Geometry check sheet. Reference: the model listing, model coordinates, mm. Give positions to 0.01 mm unless a question says otherwise; leave off trailing zeros. Write each loop counter-clockwise with the first axis right and the second up, starting at its lowest first coordinate (ties: lowest second). Pieces come first, ordered by that corner, then holes. Notation, with made-up numbers: (66.5, -29) - (116.5, -29) arc R21 cw to (116.5, -25) - close; hole circle Ø11 at (2.5, -10). An arc over 180 degrees is marked (long way). Use a Markdown table: item, result.
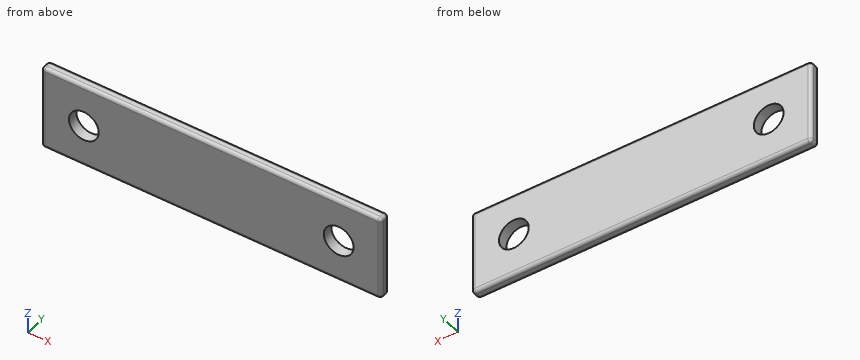
Autodesk Inventor part; units mm, degrees
ref_plane "YZ Plane" through (0, 0, 0) normal (1, 0, 0) x (0, 1, 0)
ref_plane "XZ Plane" through (0, 0, 0) normal (0, 1, 0) x (-1, 0, 0)
ref_plane "XY Plane" through (0, 0, 0) normal (0, 0, 1) x (1, 0, 0)
sketch "Sketch1" plane through (0, 0, 0) normal (0, 1, 0) x (-1, 0, 0)
  line L0 (-27.8977, 8.1703) -> (22.9023, 8.1703)
  line L1 (22.9023, 8.1703) -> (22.9023, -4.5297)
  line L2 (22.9023, -4.5297) -> (-27.8977, -4.5297)
  line L3 (-27.8977, -4.5297) -> (-27.8977, 8.1703)
  point P0 (0, 0)
  dimension "d0" = 50.8
  dimension "d1" = 12.7
extrude "Extrusion1" add sketch "Sketch1" along normal blind 1.5875
sketch "Sketch2" plane through (0, 1.5875, 0) normal (0, 1, 0) x (1, 0, 0)
  line L0 (27.8977, -8.1703) -> (27.8977, 4.5297)
  line L1 (27.8977, 4.5297) -> (-22.9023, 4.5297)
  line L2 (-22.9023, 4.5297) -> (-22.9023, -8.1703)
  circle A0 centre (-16.5523, -1.8203) radius 2.2225
  circle A1 centre (21.5477, -1.8203) radius 2.2225
  point P0 (0, 0)
  dimension "d4" = 4.445
  dimension "d5" = 6.35
  dimension "d6" = 4.445
  dimension "d7" = 6.35
  dimension "d8" = 6.35
  dimension "d9" = 6.35
extrude "Extrusion2" cut sketch "Sketch2" against normal blind 1.5875
fillet "Fillet1" radius 0.508 12 edges at (2.4977, 1.5875, 8.1703) (-22.9023, 0, 1.8203) (-22.9023, 0.7937, 8.1703) (-22.9023, 1.5875, 1.8203) (-22.9023, 0.7937, -4.5297) (2.4977, 0, -4.5297) (2.4977, 1.5875, -4.5297) (27.8977, 0.7937, -4.5297) (27.8977, 0, 1.8203) (27.8977, 1.5875, 1.8203) (27.8977, 0.7937, 8.1703) (2.4977, 0, 8.1703)
properties part number "4 hole long poly"
1) Material ranges on L1, parallel to X at y = 0.1, z = 3.75; L2, parallel to X at y = 1.5, z = 2; L3, parallel to Y at x = -4.5, z = 7.75, recorded low to high. Write a range as from..to.
Working result:
| item | result |
|---|---|
| L1 | x = -22.7..-17.65, -15.45..20.45, 22.65..27.69 |
| L2 | x = -22.68..-18.77, -14.34..19.33, 23.76..27.67 |
| L3 | y = 0.01..1.58 |
2) Section check C-C on z = 0.5. Record the boundary of the cut face in (x, y), then the cut area to 3 significant figures.
Working result:
| item | result |
|---|---|
| outline | (-22.9, 0.51) arc R0.51 ccw to (-22.39, 0) - (-18.34, 0) - (-18.34, 1.59) - (-22.39, 1.59) arc R0.51 ccw to (-22.9, 1.08) - close; (-14.76, 0) - (19.76, 0) - (19.76, 1.59) - (-14.76, 1.59) - close; (23.34, 0) - (27.39, 0) arc R0.51 ccw to (27.9, 0.51) - (27.9, 1.08) arc R0.51 ccw to (27.39, 1.59) - (23.34, 1.59) - close |
| area | 69.1 mm² |
3) Section check A-A on z = 3.25. Record the boundary of the cut face in (x, y), then the cut area to 3 significant figures.
Working result:
| item | result |
|---|---|
| outline | (-22.9, 0.51) arc R0.51 ccw to (-22.39, 0) - (-18.25, 0) - (-18.25, 1.59) - (-22.39, 1.59) arc R0.51 ccw to (-22.9, 1.08) - close; (-14.85, 0) - (19.85, 0) - (19.85, 1.59) - (-14.85, 1.59) - close; (23.25, 0) - (27.39, 0) arc R0.51 ccw to (27.9, 0.51) - (27.9, 1.08) arc R0.51 ccw to (27.39, 1.59) - (23.25, 1.59) - close |
| area | 69.6 mm² |
4) Section check B-B on x = 21.5. Record the boundary of the cut face in (y, z), then the cut area to 3 significant figures.
Working result:
| item | result |
|---|---|
| outline | (0, -4.02) arc R0.51 ccw to (0.51, -4.53) - (1.08, -4.53) arc R0.51 ccw to (1.59, -4.02) - (1.59, -0.4) - (0, -0.4) - close; (0, 4.04) - (1.59, 4.04) - (1.59, 7.66) arc R0.51 ccw to (1.08, 8.17) - (0.51, 8.17) arc R0.51 ccw to (0, 7.66) - close |
| area | 12.9 mm² |
